The drawing under review shows one solid part. Ordinate dimensions are in mm from its lowest x, y, z. Coordinates: 2 decimals unless noted, no trailing zeros. Loops run counter-clockwise (first coordinate to the right, second up) from the corner with the lowest first, then second, coordinate; pieces in that order, holes last. Notation, with made-up numbers: M 60.25,13.5 L 87.25,13.5 A22 cw 87.25,23.5 Z; hole C 38,-30 d2. An arc over 180 degrees is marked long. Put each result on its own line as item: value.
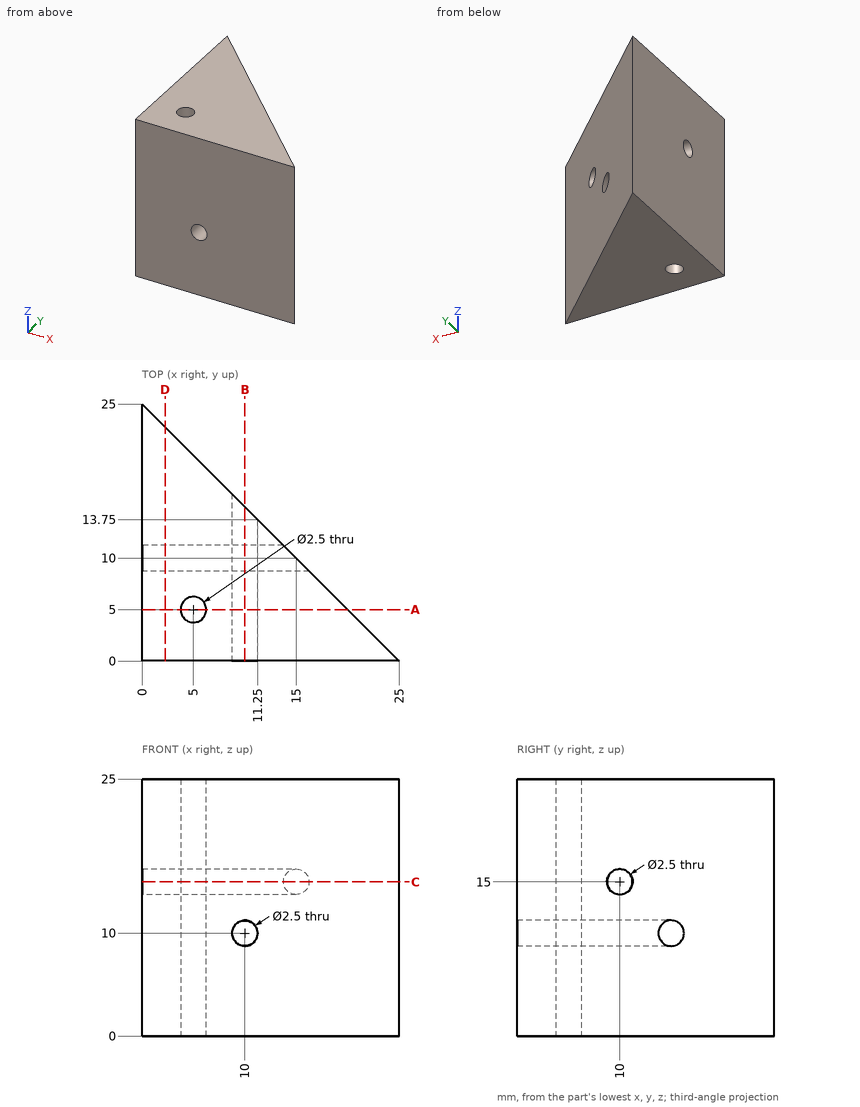
(1) Add section C-C (z = 15). Write out the cut boundary in (x, y).
Determined:
outline: M 0,0 L 25,0 L 16.25,8.75 L 0,8.75 Z; M 0,11.25 L 13.75,11.25 L 0,25 Z; hole C 5,5 d2.5
(2) Add section B-B (x = 10). Write out the cut boundary in (y, z), plus the area to 3 significant figures.
Determined:
outline: M 0,0 L 15,0 L 15,8.75 L 0,8.75 Z; M 0,11.25 L 15,11.25 L 15,25 L 0,25 Z; hole C 10,15 d2.5
area: 333 mm^2
(3) For pin 1 (1 mm diameter, centred on x = 4.5, z = 22, fed in from +Y); pin 2 (2 mm diameter, centred on y = 10, z = 15, fed in from +X); pin 3 (2 mm diameter, centred on x = 10.5, z = 21.5, fed in from +Y); pin 4 (2 mm diameter, centred on x = 2.5, z = 18, fed in from +Y), all flat-tipped, find the tip position at first contact; note any pin that passes through.
Determined:
pin 1: stops at y = 21
pin 2: passes through
pin 3: stops at y = 15.5
pin 4: stops at y = 23.5
(4) Add section A-A (y = 5). Write out the cut boundary in (x, z).
Determined:
outline: M 0,0 L 3.75,0 L 3.75,25 L 0,25 Z; M 6.25,0 L 20,0 L 20,25 L 6.25,25 Z; hole C 10,10 d2.5
(5) Wall thickness on line 1 along Z through (x, y) = (10, 13.5); line 2 along Y through (x, z) = (4.25, 15); line 3 along Y through (x, z) = (5, 15): over which ranges is each line inside the solid? List them lowest first. Write a range as [from, to].
Determined:
line 1: z = [0, 8.75], [11.25, 25]
line 2: y = [0, 4], [6, 8.75], [11.25, 20.75]
line 3: y = [0, 3.75], [6.25, 8.75], [11.25, 20]
(6) Add section D-D (x = 2.25). Write out the cut boundary in (y, z).
Determined:
outline: M 0,0 L 22.75,0 L 22.75,25 L 0,25 Z; hole C 10,15 d2.5
